from build123d import *

# Parameters (mm, degrees)
SKETCH1_R           = 10
SKETCH1_R_2         = 5.5
BOSS_EXTRUDE1_DEPTH = 2
SKETCH3_R           = 3
BOSS_EXTRUDE2_DEPTH = 12
SKETCH4_R           = 10
SKETCH4_R_2         = 3
BOSS_EXTRUDE3_DEPTH = 2
CHAMFER2_SIZE       = 1
CHAMFER4_SIZE       = 0.5
CUT_EXTRUDE1_REACH  = 6
SKETCH5_R           = 0.75
SKETCH6_R           = 6.25
SKETCH6_R_2         = 5.5
BOSS_EXTRUDE4_DEPTH = 26
CUT_EXTRUDE2_REACH  = 32
SKETCH7_R           = 0.75
SKETCH8_R           = 16.614534325
CUT_EXTRUDE3_DEPTH  = 12


with BuildPart() as part:
    # Sketch1 → Boss-Extrude1 (new body)
    with BuildSketch(Plane.XY):
        Circle(SKETCH1_R)
        Circle(SKETCH1_R_2, mode=Mode.SUBTRACT)
    extrude(amount=BOSS_EXTRUDE1_DEPTH)



with BuildPart() as body_2:
    # Sketch3 → Boss-Extrude2 (new body)
    with BuildSketch(Plane(origin=(0, 0, 0), x_dir=(-1, 0, 0), z_dir=(0, 0, -1))):
        Circle(SKETCH3_R)
    extrude(amount=BOSS_EXTRUDE2_DEPTH)


with BuildPart() as part_1:
    add(part.part)

    add(body_2.part)  # Boss-Extrude3 merges body 2
    # Sketch4 → Boss-Extrude3 (add)
    with BuildSketch(Plane(origin=(0, 0, 0), x_dir=(-1, 0, 0), z_dir=(0, 0, -1))):
        Circle(SKETCH4_R)
        Circle(SKETCH4_R_2, mode=Mode.SUBTRACT)
    extrude(amount=BOSS_EXTRUDE3_DEPTH)

    # Chamfer2
    chamfer2_edges = [part_1.edges().sort_by_distance(p)[0] for p in [
        (3, 0, -2),
    ]]
    chamfer(chamfer2_edges, length=CHAMFER2_SIZE)

    # Chamfer4
    chamfer4_edges = [part_1.edges().sort_by_distance(p)[0] for p in [
        (3, 0, -12),
    ]]
    chamfer(chamfer4_edges, length=CHAMFER4_SIZE)

    # Sketch5 → Cut-Extrude1 (cut, up to next)
    with BuildSketch(Plane(origin=(0, 0, -2), x_dir=(-1, 0, 0), z_dir=(0, 0, -1)), mode=Mode.PRIVATE) as cut_extrude1_sk1:
        with Locations((-8.5, 0)):
            Circle(SKETCH5_R)
    cut_extrude1_tool1 = extrude(cut_extrude1_sk1.sketch, amount=-CUT_EXTRUDE1_REACH, mode=Mode.PRIVATE) & part_1.part
    add(cut_extrude1_tool1.solids().sort_by_distance((8.5, 0, -2))[0], mode=Mode.SUBTRACT)
    # Sketch5 → Cut-Extrude1 (cut, up to next)
    with BuildSketch(Plane(origin=(0, 0, -2), x_dir=(-1, 0, 0), z_dir=(0, 0, -1)), mode=Mode.PRIVATE) as cut_extrude1_sk2:
        with Locations((8.5, 0)):
            Circle(SKETCH5_R)
    cut_extrude1_tool2 = extrude(cut_extrude1_sk2.sketch, amount=-CUT_EXTRUDE1_REACH, mode=Mode.PRIVATE) & part_1.part
    add(cut_extrude1_tool2.solids().sort_by_distance((-8.5, 0, -2))[0], mode=Mode.SUBTRACT)

    # Sketch6 → Boss-Extrude4 (add)
    with BuildSketch(Plane.XY.offset(2)):
        Circle(SKETCH6_R)
        Circle(SKETCH6_R_2, mode=Mode.SUBTRACT)
    extrude(amount=BOSS_EXTRUDE4_DEPTH)

    # Sketch7 → Cut-Extrude2 (cut, up to next)
    with BuildSketch(Plane(origin=(0, 0, -2), x_dir=(-1, 0, 0), z_dir=(0, 0, -1)), mode=Mode.PRIVATE) as cut_extrude2_sk1:
        with Locations((0, 7.5)):
            Circle(SKETCH7_R)
    cut_extrude2_tool1 = extrude(cut_extrude2_sk1.sketch, amount=-CUT_EXTRUDE2_REACH, mode=Mode.PRIVATE) & part_1.part
    add(cut_extrude2_tool1.solids().sort_by_distance((0, 7.5, -2))[0], mode=Mode.SUBTRACT)
    # Sketch7 → Cut-Extrude2 (cut, up to next)
    with BuildSketch(Plane(origin=(0, 0, -2), x_dir=(-1, 0, 0), z_dir=(0, 0, -1)), mode=Mode.PRIVATE) as cut_extrude2_sk2:
        with Locations((6.495190528, -3.75)):
            Circle(SKETCH7_R)
    cut_extrude2_tool2 = extrude(cut_extrude2_sk2.sketch, amount=-CUT_EXTRUDE2_REACH, mode=Mode.PRIVATE) & part_1.part
    add(cut_extrude2_tool2.solids().sort_by_distance((-6.495191, -3.75, -2))[0], mode=Mode.SUBTRACT)
    # Sketch7 → Cut-Extrude2 (cut, up to next)
    with BuildSketch(Plane(origin=(0, 0, -2), x_dir=(-1, 0, 0), z_dir=(0, 0, -1)), mode=Mode.PRIVATE) as cut_extrude2_sk3:
        with Locations((-6.495190528, -3.75)):
            Circle(SKETCH7_R)
    cut_extrude2_tool3 = extrude(cut_extrude2_sk3.sketch, amount=-CUT_EXTRUDE2_REACH, mode=Mode.PRIVATE) & part_1.part
    add(cut_extrude2_tool3.solids().sort_by_distance((6.495191, -3.75, -2))[0], mode=Mode.SUBTRACT)

    # Sketch8 → Cut-Extrude3 (cut)
    with BuildSketch(Plane(origin=(0, 0, -12), x_dir=(-1, 0, 0), z_dir=(0, 0, -1))):
        Circle(SKETCH8_R)
    extrude(amount=-CUT_EXTRUDE3_DEPTH, mode=Mode.SUBTRACT)


solid = part_1.part
For this review, take the finished solid that the model builds, in its own axes (mm). A direction names the side the tool comes from. Coordinates: 2 decimals unless noted, no trailing zeros. Order: outer loops, then holes, each group sorted by start corner. A loop starts at its lowest first (then second) coordinate and runs counter-clockwise, first axis right, second up. Notation, with made-up numbers: (-32, -18) - (-23, -18) arc R15 ccw to (-23, -11) - close; hole circle Ø6 at (33.25, -8.5). An arc over 180 degrees is marked (long way). Answer as CSV lines item,"result". Start each with the question number.
1) To check wall thickness, follow line 1 along Y through (x, z) = (0, 25.5); line 2 along Z through (x, y) = (-4.5, -4.5); line 3 along X through (y, z) = (3.75, 5.75). State the ranges of each line that lie inside material, in increasing order. Write a range as [from, to].
2) Machinability: for faces 1 (the cylindrical face through (5.96, 1.88, 14.82)), 2 (the cylindrical face through (0.55, 8.01, 0.99)), which of the approach directions +Z, -Z, +X, -X, +Y, -Y give a long, thin tool a straight path to every point of the face, cutting with its end or side? Answer none if there is none.
3) Add section D-D (z = 24.25). State the section outline as (x, y) points, then the cut area to 3 significant figures.
4) Add section C-C (x = -8.5). State the section outline as (y, z) points, then the cut area to 3 significant figures.
5) Add section B-B (x = 0). State the section outline as (y, z) points, then the cut area to 3 significant figures.
6) Add section A-A (y = 0). State the section outline as (x, z) points.
7) Draft analysis for pull direction Y (two halves, no side actions). For faces 3 (the flat face through (4, 5, 2)), 4 (the cylindrical face through (-2.17, -9.76, 0.99)), 5 (the cylindrical face through (-1.19, -5.37, 13.8)), state which applies: +Y half, -Y half, draft (parallel to the pull), parting line (faces both ways), or undercut.
8) Insertion check: P1, Ø1, axis at y = -3.5, z = 14.5, coming from the -X side; P2, Ø2, axis at x = 5.5, z = 4.5, coming from the +Y side; P3, Ø5, axis at x = 7.5, z = 13, coming from the -Y side. Each pin has a flat end and moves straight along its axis. Give the tip position at first contact, or say it passes through.
Result:
1,line 1,"[-6.25, -5.5], [5.5, 6.25]"
1,line 2,"[0, 2]"
1,line 3,"[-5, -4.02], [4.02, 5]"
2,face 1,"+Z"
2,face 2,"+Z, -Z"
3,outline,"circle Ø12.5 at (0, 0); hole circle Ø11 at (0, 0)"
3,area,"27.7 mm^2"
4,outline,"(-5.27, 0) - (-0.75, 0) - (-0.75, 2) - (-5.27, 2) - close; (0.75, 0) - (5.27, 0) - (5.27, 2) - (0.75, 2) - close"
4,area,"18.1 mm^2"
5,outline,"(-10, 0) - (-5.5, 0) - (-5.5, 28) - (-6.25, 28) - (-6.25, 2) - (-10, 2) - close; (5.5, 0) - (6.75, 0) - (6.75, 2) - (6.25, 2) - (6.25, 28) - (5.5, 28) - close; (8.25, 0) - (10, 0) - (10, 2) - (8.25, 2) - close"
5,area,"54.0 mm^2"
6,outline,"(-10, 0) - (-9.25, 0) - (-9.25, 2) - (-10, 2) - close; (-7.75, 0) - (-5.5, 0) - (-5.5, 28) - (-6.25, 28) - (-6.25, 2) - (-7.75, 2) - close; (5.5, 0) - (7.75, 0) - (7.75, 2) - (6.25, 2) - (6.25, 28) - (5.5, 28) - close; (9.25, 0) - (10, 0) - (10, 2) - (9.25, 2) - close"
7,face 3,"draft"
7,face 4,"parting line"
7,face 5,"undercut"
8,P1,"x = -5.48"
8,P2,"y = 4.34"
8,P3,"y = -3.75"
